Autodesk Inventor part; units mm, degrees
ref_plane "YZ Plane" through (0, 0, 0) normal (1, 0, 0) x (0, 1, 0)
ref_plane "XZ Plane" through (0, 0, 0) normal (0, 1, 0) x (-1, 0, 0)
ref_plane "XY Plane" through (0, 0, 0) normal (0, 0, 1) x (1, 0, 0)
sketch "Sketch1" plane through (0, 0, 0) normal (0, 1, 0) x (-1, 0, 0)
  line L0 (-25.4, -25.4) -> (25.4, -25.4)
  line L1 (25.4, -25.4) -> (25.4, 25.4)
  line L2 (25.4, 25.4) -> (-25.4, 25.4)
  line L3 (-25.4, 25.4) -> (-25.4, -25.4)
  line L4 (-25.4, -25.4) -> (25.4, 25.4) construction
  line L5 (25.4, -25.4) -> (-25.4, 25.4) construction
  line L6 (26.9875, 26.9875) -> (26.9875, -26.9875)
  line L7 (26.9875, -26.9875) -> (-26.9875, -26.9875)
  line L8 (-26.9875, -26.9875) -> (-26.9875, 26.9875)
  line L9 (-26.9875, 26.9875) -> (26.9875, 26.9875)
  point P0 (0, 0)
  dimension "d0" = 50.8
  dimension "d1" = 50.8
  dimension "d2" = -1.5875
extrude "Extrusion1" add sketch "Sketch1" along normal mid plane 43.18
sketch "Sketch2" plane through (-25.4, 21.59, 25.4) normal (0, 0, -1) x (-1, 0, 0)
  circle A0 centre (-25.4, -21.59) radius 7.747
  dimension "d5" = 15.494
extrude "Extrusion2" cut sketch "Sketch2" along normal through all both and the other way through all
properties part number "Container"
Geometry: final body of the model. Coordinates: model frame, mm. A direction names the side the tool comes from. Coordinates: 2 decimals unless noted, no trailing zeros. Loops run counter-clockwise (first coordinate to the right, second up) from the corner with the lowest first, then second, coordinate; pieces in that order, holes last. Notation, with made-up numbers: M -20,-39 L 21,-39 A14 ccw 21,-31 Z; hole C 0,35.25 d8. An arc over 180 degrees is marked long. One line per item, written item: value. Start each with the question number.
1) Cut plane B-B (z = -4). Return loops of the section in (x, y), then the cut area to 3 significant figures.
2) Pin query (flat end, axial travel): P1, Ø12.5, axis at x = 0, y = 0, coming from the -Z side. Return the tip coordinate at first contact, or that it passes through.
3) Material intervals for L1, parallel to X at y = -17.5, z = -19.5; L2, parallel to Y at x = 0, z = 26.6, sorted ascending. Write a range as from..to.
4) Cut plane D-D (x = -18). Return loops of the section in (y, z), then the cut area to 3 significant figures.
5) Draft query along X for faces 3 (the flat face through (26.988, 0, 0)), 4 (the flat face through (6.4, -5.1, 26.988)), 5 (the cylindrical face through (-4.165, 6.532, 26.183)), 6 (the flat face through (-26.988, 0, 0)). Return one class per face: released by +X, released by -X, zero draft, split by the parting line, or undercut.
6) Cut plane C-C (y = 0). Return loops of the section in (x, z), then the cut area to 3 significant figures.
7) Reachability of faces 1 (the flat face through (0, -10, -25.4)), 2 (the flat face through (2, 21.59, -26)) from +Z, -Z, +X, -X, +Y, -Y: full face, straight path, thin tool, end or side. Return the list, or none.
8) Cut plane A-A (x = 0). Return loops of the section in (y, z).
Evaluation:
1. outline: M -26.99,-21.59 L -25.4,-21.59 L -25.4,21.59 L -26.99,21.59 Z; M 25.4,-21.59 L 26.99,-21.59 L 26.99,21.59 L 25.4,21.59 Z
1. area: 137 mm^2
2. P1: through
3. L1: -26.99..-25.4, 25.4..26.99
3. L2: -21.59..-7.75, 7.75..21.59
4. outline: M -21.59,-26.99 L 21.59,-26.99 L 21.59,-25.4 L -21.59,-25.4 Z; M -21.59,25.4 L 21.59,25.4 L 21.59,26.99 L -21.59,26.99 Z
4. area: 137 mm^2
5. face 3: released by +X
5. face 4: zero draft
5. face 5: undercut
5. face 6: released by -X
6. outline: M -26.99,-26.99 L -7.75,-26.99 L -7.75,-25.4 L -25.4,-25.4 L -25.4,25.4 L -7.75,25.4 L -7.75,26.99 L -26.99,26.99 Z; M 7.75,-26.99 L 26.99,-26.99 L 26.99,26.99 L 7.75,26.99 L 7.75,25.4 L 25.4,25.4 L 25.4,-25.4 L 7.75,-25.4 Z
6. area: 283 mm^2
7. face 1: +Y, -Y
7. face 2: +Z, -Z, +X, -X, +Y
8. outline: M -21.59,-26.99 L -7.75,-26.99 L -7.75,-25.4 L -21.59,-25.4 Z; M -21.59,25.4 L -7.75,25.4 L -7.75,26.99 L -21.59,26.99 Z; M 7.75,-26.99 L 21.59,-26.99 L 21.59,-25.4 L 7.75,-25.4 Z; M 7.75,25.4 L 21.59,25.4 L 21.59,26.99 L 7.75,26.99 Z
